```python
from build123d import *

# Parameters (mm, degrees)
SKETCH1_R               = 22.5
SKETCH1_R_2             = 2.55
BOSS_EXTRUDE1_DEPTH     = 7.3
SKETCH2_R               = 1.525
CUT_EXTRUDE1_DEPTH      = 3.4
CUT_EXTRUDE2_DEPTH      = 33.646439316
CUT_EXTRUDE2_DEPTH_BACK = 33.646439316
SKETCH3_R               = 2.55
SKETCH3_R_2             = 1.65
CHAMFER7_SIZE           = 1
CHAMFER8_SIZE           = 3
CUT_EXTRUDE3_DEPTH      = 2
BOSS_EXTRUDE2_START     = -5.3
BOSS_EXTRUDE2_DEPTH     = 5.3


with BuildPart() as part:
    # Sketch1 → Boss-Extrude1 (new body)
    with BuildSketch(Plane.XY):
        Circle(SKETCH1_R)
        Circle(SKETCH1_R_2, mode=Mode.SUBTRACT)
    extrude(amount=BOSS_EXTRUDE1_DEPTH)

    # Sketch2 → Cut-Extrude1 (cut)
    with BuildSketch(Plane(origin=(0, 0, 0), x_dir=(-1, 0, 0), z_dir=(0, 0, -1))):
        with Locations((-18.85, 0)):
            Circle(SKETCH2_R)
        with Locations((-5.824970344, 17.927415332)):
            Circle(SKETCH2_R)
        with Locations((15.249970344, 11.079752006)):
            Circle(SKETCH2_R)
        with Locations((15.249970344, -11.079752006)):
            Circle(SKETCH2_R)
        with Locations((-5.824970344, -17.927415332)):
            Circle(SKETCH2_R)
    extrude(amount=-CUT_EXTRUDE1_DEPTH, mode=Mode.SUBTRACT)

    # Sketch3 → Cut-Extrude2 (cut, two sides: drawn at the far end of the back side and taken through both)
    with BuildSketch(Plane(origin=(0, 0, 0), x_dir=(-1, 0, 0), z_dir=(0, 0, -1)).offset(-CUT_EXTRUDE2_DEPTH_BACK)):
        with Locations(Location((0, 0, 0), (0, 0, 180))):
            Circle(SKETCH3_R)
        with Locations((-10.9375, 0)):
            Circle(SKETCH3_R_2)
        with Locations((-3.395324226, 10.449733473)):
            Circle(SKETCH3_R_2)
        with Locations((8.873623376, 6.505843285)):
            Circle(SKETCH3_R_2)
        with Locations((8.914074226, -6.381348371)):
            Circle(SKETCH3_R_2)
        with Locations((-3.329873376, -10.402180647)):
            Circle(SKETCH3_R_2)
    extrude(amount=CUT_EXTRUDE2_DEPTH + CUT_EXTRUDE2_DEPTH_BACK, mode=Mode.SUBTRACT)

    # Chamfer7
    chamfer7_edges = [part.edges().sort_by_distance(p)[0] for p in [
        (-22.5, 0, 0),
    ]]
    chamfer(chamfer7_edges, length=CHAMFER7_SIZE)

    # Chamfer8
    chamfer8_edges = [part.edges().sort_by_distance(p)[0] for p in [
        (-22.5, 0, 7.3),
    ]]
    chamfer(chamfer8_edges, length=CHAMFER8_SIZE)

    # Sketch8 → Cut-Extrude3 (cut)
    with BuildSketch(Plane(origin=(0, 0, 0), x_dir=(-1, 0, 0), z_dir=(0, 0, -1))):
        with BuildLine():
            Line((-5.65, -6.549809158), (-5.65, 6.549809158))
            ThreePointArc((-5.65, 6.549809158), (8.65, 0), (-5.65, -6.549809158))
        make_face()
    extrude(amount=-CUT_EXTRUDE3_DEPTH, mode=Mode.SUBTRACT)

    # Sketch10 → Boss-Extrude2 (add)
    with BuildSketch(Plane.XY.offset(7.3).offset(BOSS_EXTRUDE2_START)):
        with BuildLine():
            Line((-2.3, -1.101135777), (-2.3, 1.101135777))
            ThreePointArc((-2.3, 1.101135777), (-2.55, 0), (-2.3, -1.101135777))
        make_face()
    extrude(amount=BOSS_EXTRUDE2_DEPTH)


solid = part.part
```
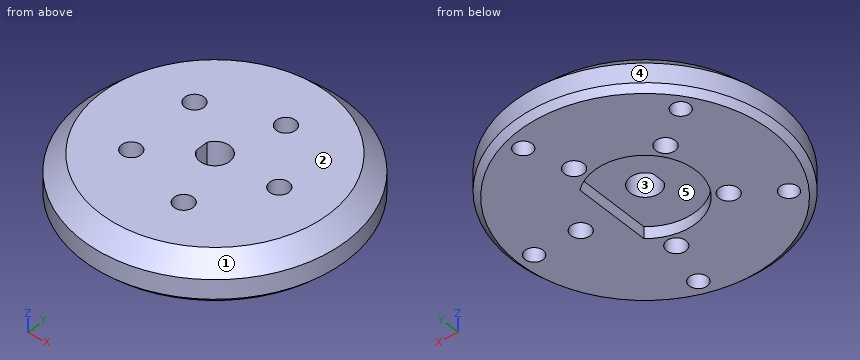
Model file for the job. Use its own axes, mm. Face numbers are marked on the shaded views. A direction names the side the tool comes from. Coordinates: 2 decimals unless noted, no trailing zeros. Loops run counter-clockwise (first coordinate to the right, second up) from the corner with the lowest first, then second, coordinate; pieces in that order, holes last. Notation, with made-up numbers: (79.25, 62) -> (116.25, 62) arc R26 ccw to (116.25, 100) -> close; hole circle Ø6 at (17.25, 69). An arc over 180 degrees is marked (long way). Answer as a JSON object with one key per item and string values.
Q1. Flat gauge pins, fed straight in: P1, Ø2.5, axis at x = -15.25, y = -11.08, coming from the -Z side; P2, Ø15.5, axis at x = 0.5, y = 1.5, coming from the -Z side; P3, Ø2, axis at y = 2.5, z = 1, coming from the -X side; P4, Ø2, axis at y = 5, z = 2, coming from the +X side. Where does each tip first touch, or does it go through?
Report:
{"P1": "stops at z = 3.4", "P2": "stops at z = 0", "P3": "stops at x = -22.45", "P4": "stops at x = 22.14"}
Q2. Cut at A-A (y = 0). State how many separate pieces and enclosed holes the cut face has, and give its area (3 significant figures).
Report:
{"separate pieces": "3", "enclosed holes": "0", "area": "230 mm2"}
Q3. 3-axis set-ups, long thin cutter, end or side, ignore diameter. For the marked faces 4 and 5: which of +Z, -Z, +X, -X, +Y, -Y reach the whole face in a straight line?
Report:
{"face 4": "+Z, -Z", "face 5": "-Z"}
Q4. Cut at B-B (x = 0). List the corners of the cut face in (y, z), and give its area (3 significant figures).
Report:
{"outline": "(-22.5, 1) -> (-21.5, 0) -> (-8.65, 0) -> (-8.65, 2) -> (-2.55, 2) -> (-2.55, 7.3) -> (-19.5, 7.3) -> (-22.5, 4.3) -> close; (2.55, 2) -> (8.65, 2) -> (8.65, 0) -> (21.5, 0) -> (22.5, 1) -> (22.5, 4.3) -> (19.5, 7.3) -> (2.55, 7.3) -> close", "area": "257 mm2"}
Q5. Pull direction X, two halves, no side cores. Call the marked faces 1, 2 and 3: released by +X, released by -X, zero draft, split by the parting line, or undercut.
Report:
{"face 1": "split by the parting line", "face 2": "zero draft", "face 3": "undercut"}
Q6. Probe probe 1 along Y at (x, z) = (-14, 2.5); probe 2 along X at (y, z) = (11, 3); probe 3 along Y at (x, z) = (2, 6.5). List the from-to ranges inside material, lowest first.
Report:
{"probe 1": "y = -17.61 to -11.95, -10.21 to 10.21, 11.95 to 17.61", "probe 2": "x = -19.63 to -16.77, -13.73 to 1.84, 4.95 to 19.63", "probe 3": "y = -20.2 to -11.38, -9.43 to -1.58, 1.58 to 9.57, 11.33 to 20.2"}
